```python
from build123d import *


with BuildPart() as part:
    # revolution body → Revolve1 (revolve)
    with BuildSketch(Plane.XY, mode=Mode.PRIVATE) as revolve1_sk:
        with BuildLine():
            Line((-67.034317062, 8.819371739), (-54.034317062, 8.819371739))
            add(Edge.make_bspline(
                [(-54.034317062, 8.819371739), (-45.639917935, 8.716149455), (-46.425076057, 15.031715968), (-39.034317062, 15.169371739)],
                knots=[0, 0, 0, 0, 1, 1, 1, 1], degree=3))
            Line((-39.034317062, 15.169371739), (29.265682938, 15.169371739))
            ThreePointArc((29.265682938, 15.169371739), (36.33675075, 12.24043955), (39.265682938, 5.169371739))
            Line((39.265682938, 5.169371739), (39.265682938, 2.469371739))
            Line((39.265682938, 2.469371739), (-68.034317062, 2.469371739))
            Line((-68.034317062, 2.469371739), (-68.034317062, 7.819371739))
            Line((-68.034317062, 7.819371739), (-67.034317062, 8.819371739))
        make_face()
    revolve(revolve1_sk.sketch.rotate(Axis((-68.034317062, 2.469371739, 0), (1, 0, 0)), 90), axis=Axis((-68.034317062, 2.469371739, 0), (1, 0, 0)))


solid = part.part
```
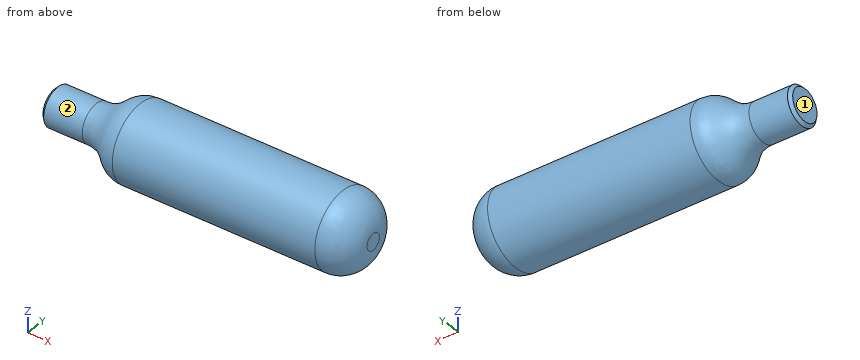
Geometry check sheet. Reference: the model listing, model coordinates, mm. Face numbers are marked on the shaded views. A direction names the side the tool comes from. Round coordinates to 2 decimals unless told otherwise and drop trailing zeros. Order: outer loops, then holes, each group sorted by start corner. A loop starts at its lowest first (then second) coordinate and runs counter-clockwise, first axis right, second up. Notation, with made-up numbers: M 86.25,-14 L 109.25,-14 A21 ccw 109.25,4 Z; hole C 24,53.5 d5. An arc over 180 degrees is marked long. Answer as CSV lines item,"result".
1) Sectioned sample at A-A on x = -7.5. Record the cut outline in (y, z).
Entries:
outline,"C 2.47,0 d25.4"
2) Gauge pin test, flat ends, axial feed: pin 1 Ø8 at (y, z) = (-0.5, 8.5) entering from -X; pin 2 Ø2 at (x, y) = (7, 5) entering from +Z; pin 3 Ø1.5 at (x, y) = (-51, 3.5) entering from +Z; pin 4 Ø10 at (x, z) = (-54.5, 7.5) entering from -Y. Record the tip position at first contact, or that the pin passes through.
Entries:
pin 1,"x = -68.03"
pin 2,"z = 12.61"
pin 3,"z = 6.8"
pin 4,"y = -3.37"
3) Thickness scan on probe 1 along Y at (x, z) = (-23, 0.25); probe 2 along X at (y, z) = (9.75, 7.5); probe 3 along Y at (x, z) = (25, 2.25). Record the ranges inside material, lowest first. Write a range as [from, to].
Entries:
probe 1,"[-10.23, 15.17]"
probe 2,"[-45, 35.58]"
probe 3,"[-10.03, 14.97]"
4) Tool access check on the marked faces 1 and 2. Record the directions out of +Z, -Z, +X, -X, +Y, -Y that give a thin tool (end or side, any length) a straight path to the whole face; none if there is none.
Entries:
face 1,"+Z, -Z, -X, +Y, -Y"
face 2,"-X"
